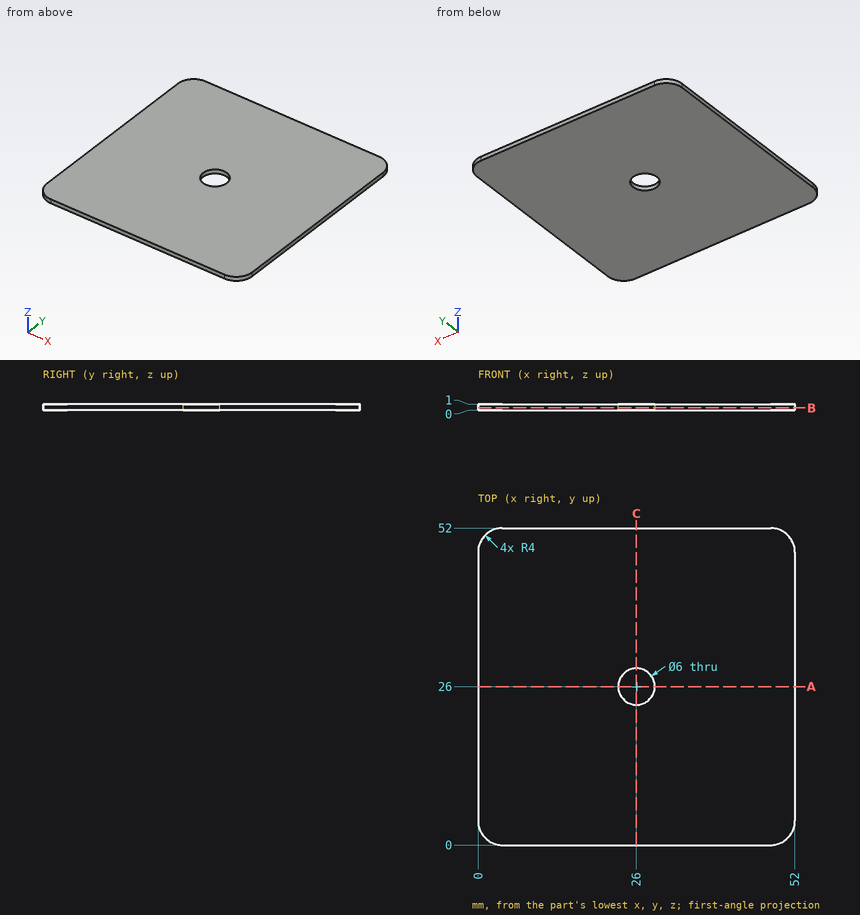
Here's the drawing with two shaded views (mm, measured from the low corner). I have some questions. Give positions to 0.01 mm unless a question says otherwise; leave off trailing zeros. Loops run counter-clockwise (first coordinate to the right, second up) from the corner with the lowest first, then second, coordinate; pieces in that order, holes last. Notation, with made-up numbers: M 57.25,81 L 75.25,81 A20 ccw 75.25,113 Z; hole C 85.5,73 d6. An arc over 180 degrees is marked long. Use one line per item in the form item = value. Start each with the question number.
Q1. I need wall thicknesses on line 1 along Y through (x, z) = (26, 0.8); line 2 along X through (y, z) = (48.5, 0.75); line 3 along Y through (x, z) = (49.5, 0.3). Which ranges of each line are inside material? Lowest first, please.
Q2. If we section it at A-A (y = 26): Write out the boundary of the cut face in (x, z).
Q3. If we section it at B-B (z = 0.35): Write out the boundary of the cut face in (x, y).
Taken from the geometry:
q1.line_1 = 0 to 23, 29 to 52
q1.line_2 = 0.03 to 51.97
q1.line_3 = 0.29 to 51.71
q2.outline = M 0,0 L 23,0 L 23,1 L 0,1 Z; M 29,0 L 52,0 L 52,1 L 29,1 Z
q3.outline = M 0,4 A4 ccw 4,0 L 48,0 A4 ccw 52,4 L 52,48 A4 ccw 48,52 L 4,52 A4 ccw 0,48 Z; hole C 26,26 d6
